Design review of the part built by this model. Coordinates are the model's own, in mm. A direction names the side the tool comes from. Coordinates: 2 decimals unless noted, no trailing zeros. Write each loop counter-clockwise with the first axis right and the second up, starting at its lowest first coordinate (ties: lowest second). Pieces come first, ordered by that corner, then holes. Notation, with made-up numbers: (46, 33) - (79, 33) arc R16 ccw to (79, 49) - close; hole circle Ø9 at (63.5, -36). An arc over 180 degrees is marked (long way). Answer as a JSON object with one key per item and string values.
```python
from build123d import *

# Parameters (mm, degrees)
SKIZZE1_R                       = 40
AUFSATZ_LINEAR_AUSTRAGEN1_DEPTH = 15
SKIZZE2_W                       = 30
SKIZZE2_H                       = 65
SKIZZE2_W_2                     = 20
AUFSATZ_LINEAR_AUSTRAGEN2_DEPTH = 67


with BuildPart() as part:
    # Skizze1 → Aufsatz-Linear austragen1 (new body)
    with BuildSketch(Plane(origin=(0, 0, 0), x_dir=(1, 0, 0), z_dir=(0, 1, 0))):
        with BuildLine():
            Line((-95.5, 40), (-95.5, -40))
            Line((-95.5, -40), (55.5, -40))
            ThreePointArc((55.5, -40), (15.5, 0), (55.5, 40))
            Line((55.5, 40), (-95.5, 40))
        make_face()
        with Locations((55.5, 0)):
            Circle(SKIZZE1_R)
        with BuildLine():
            Line((95.5, 40), (55.5, 40))
            ThreePointArc((55.5, 40), (83.784271247, 28.284271247), (95.5, 0))
            Line((95.5, 0), (95.5, 40))
        make_face()
        with BuildLine():
            ThreePointArc((95.5, 0), (83.784271247, -28.284271247), (55.5, -40))
            Line((55.5, -40), (95.5, -40))
            Line((95.5, -40), (95.5, 0))
        make_face()
    extrude(amount=AUFSATZ_LINEAR_AUSTRAGEN1_DEPTH)

    # Skizze2 → Aufsatz-Linear austragen2 (add)
    with BuildSketch(Plane(origin=(0, 15, 0), x_dir=(1, 0, 0), z_dir=(0, 1, 0))):
        with Locations((28, 0)):
            Rectangle(SKIZZE2_W, SKIZZE2_H)
        with Locations((-34, 0)):
            Rectangle(SKIZZE2_W_2, SKIZZE2_H)
    extrude(amount=AUFSATZ_LINEAR_AUSTRAGEN2_DEPTH)


solid = part.part
```
(1) Take a section at B-B, the plane z = -1. Write out the cut boundary in (x, y), and give its area (4 significant figures).
Solved:
{"outline": "(-95.5, 0) - (95.5, 0) - (95.5, 15) - (43, 15) - (43, 82) - (13, 82) - (13, 15) - (-24, 15) - (-24, 82) - (-44, 82) - (-44, 15) - (-95.5, 15) - close", "area": "6,215 mm^2"}
(2) Tool access review of faces 1 (the face through (-44, 48, 0)), 2 (the face through (28, 48, 32.5)), 3 (the face through (-34, 48, -32.5)), 4 (the face through (13, 48, 0)), 5 (the face through (43, 48, 0)): name each direction out of +Z, -Z, +X, -X, +Y, -Y from which nothing blocks a thin tool from reaching the whole face with its end or side.
Solved:
{"face 1": "+Z, -Z, -X, +Y", "face 2": "+Z, +X, -X, +Y", "face 3": "-Z, +X, -X, +Y", "face 4": "+Z, -Z, +Y", "face 5": "+Z, -Z, +X, +Y"}
(3) Take a section at A-A, the plane y = 57.5. Write out the cut boundary in (x, z), and give its area (3 significant figures).
Solved:
{"outline": "(-44, -32.5) - (-24, -32.5) - (-24, 32.5) - (-44, 32.5) - close; (13, -32.5) - (43, -32.5) - (43, 32.5) - (13, 32.5) - close", "area": "3,250 mm^2"}
(4) To check wall thickness, follow line 1 (X direction, y = 44.5, z = 15); line 2 (Y direction, x = -4.5, z = 33); line 3 (Z direction, x = 23, y = 48.5). State the ranges of each line that lie inside material, in increasing order. Write a range as from..to.
Solved:
{"line 1": "x = -44..-24, 13..43", "line 2": "y = 0..15", "line 3": "z = -32.5..32.5"}
(5) Take a section at D-D, the plane x = 78.5. Write out the cut boundary in (y, z).
Solved:
{"outline": "(0, -40) - (15, -40) - (15, 40) - (0, 40) - close"}
(6) Take a section at C-C, the plane x = 25.5. Write out the cut boundary in (y, z).
Solved:
{"outline": "(0, -40) - (15, -40) - (15, -32.5) - (82, -32.5) - (82, 32.5) - (15, 32.5) - (15, 40) - (0, 40) - close"}
(7) For pin 1 (19.5 mm diameter, centred on y = 61, z = 8, fed in from -X); pin 2 (10 mm diameter, centred on x = -69.5, y = 22.5, fed in from -Z); pin 3 (1.5 mm diameter, centred on x = 10.5, z = 2.5, fed in from +Y); pin 4 (15 mm diameter, centred on x = 25, y = 39, fed in from +Z), all flat-tipped, find the tip position at first contact; note any pin that passes through.
Solved:
{"pin 1": "stops at x = -44", "pin 2": "passes through", "pin 3": "stops at y = 15", "pin 4": "stops at z = 32.5"}
